```python
from build123d import *

# Parameters (mm, degrees)
SKETCH1_R           = 18
BOSS_EXTRUDE3_DEPTH = 33
SKETCH12_R          = 2
CUT_EXTRUDE1_DEPTH  = 10
SKETCH13_W          = 67.899494937
SKETCH13_H          = 35
BOSS_EXTRUDE4_DEPTH = 33
SKETCH14_R          = 1.62
CUT_EXTRUDE2_DEPTH  = 10
SKETCH15_R          = 20
CUT_EXTRUDE3_DEPTH  = 79.208702146


with BuildPart() as part:
    # Sketch1 → Boss-Extrude3 (new body)
    with BuildSketch(Plane(origin=(0, 0, 0), x_dir=(1, 0, 0), z_dir=(0, 1, 0))):
        with BuildLine():
            Line((-47.308295415, 17.815966111), (20.591199522, 17.815966111))
            Line((20.591199522, 17.815966111), (20.591199522, 9.675262593))
            Line((20.591199522, 9.675262593), (10.591199522, 9.675262593))
            Line((10.591199522, 9.675262593), (10.591199522, -35.324737407))
            Line((10.591199522, -35.324737407), (2.365275891, -35.324737407))
            ThreePointArc((2.365275891, -35.324737407), (-13.358547947, -40.274484875), (-29.082371784, -35.324737407))
            Line((-29.082371784, -35.324737407), (-37.308295415, -35.324737407))
            Line((-37.308295415, -35.324737407), (-37.308295415, 9.675262593))
            Line((-37.308295415, 9.675262593), (-47.308295415, 9.675262593))
            Line((-47.308295415, 9.675262593), (-47.308295415, 17.815966111))
        make_face()
        with Locations(Location((-13.358547947, -12.824737407, 0), (0, 0, 270))):
            Circle(SKETCH1_R, mode=Mode.SUBTRACT)
    extrude(amount=BOSS_EXTRUDE3_DEPTH)

    # Sketch12 → Cut-Extrude1 (cut)
    with BuildSketch(Plane(origin=(0, 0, -17.815966111), x_dir=(-1, 0, 0), z_dir=(0, 0, -1))):
        with Locations((39.788295415, 4)):
            Circle(SKETCH12_R)
        with Locations((39.788295415, 29)):
            Circle(SKETCH12_R)
        with Locations((-13.071199522, 29)):
            Circle(SKETCH12_R)
        with Locations((-13.071199522, 4)):
            Circle(SKETCH12_R)
    extrude(amount=-CUT_EXTRUDE1_DEPTH, mode=Mode.SUBTRACT)

    # Sketch13 → Boss-Extrude4 (add)
    with BuildSketch(Plane(origin=(0, 33, 0), x_dir=(1, 0, 0), z_dir=(0, 1, 0))):
        with Locations((-13.358547947, 35.315966111)):
            Rectangle(SKETCH13_W, SKETCH13_H)
    extrude(amount=-BOSS_EXTRUDE4_DEPTH)

    # Sketch14 → Cut-Extrude2 (cut)
    with BuildSketch(Plane(origin=(0, 33, 0), x_dir=(1, 0, 0), z_dir=(0, 1, 0))):
        with Locations(Location((-25.358295415, 16.899970921, 0), (0, 0, 270))):
            Circle(SKETCH14_R)
        with Locations(Location((-1.358295415, 16.899970921, 0), (0, 0, 270))):
            Circle(SKETCH14_R)
        with Locations(Location((-25.358295415, 44.899970921, 0), (0, 0, 270))):
            Circle(SKETCH14_R)
        with Locations(Location((-1.358295415, 44.899970921, 0), (0, 0, 270))):
            Circle(SKETCH14_R)
    extrude(amount=-CUT_EXTRUDE2_DEPTH, mode=Mode.SUBTRACT)

    # Sketch15 → Cut-Extrude3 (cut, through all)
    with BuildSketch(Plane.XZ):
        with Locations(Location((-13.358547947, 12.824737407, 0), (0, 0, 270))):
            Circle(SKETCH15_R)
    extrude(amount=-CUT_EXTRUDE3_DEPTH, mode=Mode.SUBTRACT)


solid = part.part
```
Can you work these out from the model? Positions are in its coordinate system, mm. A direction names the side the tool comes from. Give positions to 0.01 mm unless a question says otherwise; leave off trailing zeros. Write each loop counter-clockwise with the first axis right and the second up, starting at its lowest first coordinate (ties: lowest second). Pieces come first, ordered by that corner, then holes. Notation, with made-up numbers: (-18.5, 80.25) - (6.5, 80.25) arc R20 ccw to (6.5, 119.25) - close; hole circle Ø4 at (46, 71.25). An arc over 180 degrees is marked (long way). Write item = value, one per line. Start each with the question number.
1. Imagine slicing it at B-B (x = -28). Please give me the cut outline in (y, z).
2. Imagine slicing it at D-D (z = -1.5). Please give me the cut outline in (x, y), and give its area (3 significant figures).
3. For pin 1 (6 mm diameter, centred on x = -28.5, y = 16.5, fed in from +Z); pin 2 (1.6 mm diameter, centred on x = -25, z = -16.5, fed in from +Y); pin 3 (4.5 mm diameter, centred on x = 13.07, y = 4, fed in from +Z); pin 4 (1.9 mm diameter, centred on x = -1.36, z = -44.9, fed in from -Y), each with a flat end and sliding along its axis, tell me the tip position at first contact or that it passes through.
4. Imagine slicing it at A-A (z = -12.5). Please give me the cut outline in (x, y), and give its area (3 significant figures).
5. Imagine slicing it at C-C (y = 4). Please give me the cut outline in (x, z).
6. On a 3-axis mill with a long thin cutter (end or side, diameter ignored), from which of +Z, -Z, +X, -X, +Y, -Y can I reach the whole of each face in a straight line? I mean faces 1 (the face through (-33, 16, 35.325)), 2 (the face through (-40, 4, -17.816)), 3 (the face through (-24.26, 28.07, -18.09)), 4 (the face through (10.591, 16, 13)). Say none if no direction works.
7. Please list where these lines run through material, in increasing order: line 1 (Z direction, x = -13.5, y = 31.5); line 2 (Z direction, x = 18, y = 3); line 3 (X direction, y = 27.5, z = 14.5).
8. Thinking about a two-plate mould opening in Y: for faces 5 (the face through (-14, 0, -17)), 6 (the face through (-24.872, 28.07, -43.355)), 7 (the face through (-40, 29, -17.816)), 8 (the face through (-25, 23, -45)), which applies, released by +Y, released by -Y, zero draft, split by the parting line, or undercut?
Worked answers:
q1.outline = (0, -52.82) - (33, -52.82) - (33, -0.8) - (0, -0.8) - close; (0, 26.45) - (33, 26.45) - (33, 36.04) - (0, 36.04) - close
q2.outline = (-37.31, 0) - (-27.32, 0) - (-27.32, 33) - (-37.31, 33) - close; (0.6, 0) - (10.59, 0) - (10.59, 33) - (0.6, 33) - close
q2.area = 660 mm2
q3.pin_1 = 37.44
q3.pin_2 = 23
q3.pin_3 = -9.68
q3.pin_4 = 0
q4.outline = (-47.31, 0) - (20.59, 0) - (20.59, 33) - (-47.31, 33) - close; hole circle Ø4 at (-39.79, 4); hole circle Ø4 at (-39.79, 29); hole circle Ø4 at (13.07, 4); hole circle Ø4 at (13.07, 29)
q4.area = 2,190 mm2
q5.outline = (-47.31, -52.82) - (20.59, -52.82) - (20.59, -9.68) - (15.07, -9.68) - (15.07, -17.82) - (11.07, -17.82) - (11.07, -9.68) - (10.59, -9.68) - (10.59, 35.32) - (2.37, 35.32) arc R27.45 ccw to (-29.08, 35.32) - (-37.31, 35.32) - (-37.31, -9.68) - (-37.79, -9.68) - (-37.79, -17.82) - (-41.79, -17.82) - (-41.79, -9.68) - (-47.31, -9.68) - close; hole circle Ø40 at (-13.36, 12.82)
q6.face_1 = +Z, -X, +Y, -Y
q6.face_2 = +Z
q6.face_3 = +Y
q6.face_4 = +Z, +X, +Y, -Y
q7.line_1 = -52.82 to -7.17, 32.82 to 40.27
q7.line_2 = -52.82 to -9.68
q7.line_3 = -37.31 to -33.29, 6.57 to 10.59
q8.face_5 = released by -Y
q8.face_6 = zero draft
q8.face_7 = undercut
q8.face_8 = released by +Y
